from build123d import *

# Parameters (mm, degrees)
SKETCH1_W          = 5
SKETCH1_H          = 15
CLAMP_PART_DEPTH   = 2.5
SKETCH1_H_2        = 1.5
CLAMP_PART_2_DEPTH = 2.5
SKETCH2_R          = 1
OUTSIDE_DEPTH      = 2


with BuildPart() as part:
    # Sketch1 → Clamp part (new body)
    with BuildSketch(Plane(origin=(0, 0, -7), x_dir=(-1, 0, 0), z_dir=(0, 0, -1))):
        with Locations((19, 34)):
            Rectangle(SKETCH1_W, SKETCH1_H)
    extrude(amount=-CLAMP_PART_DEPTH)



with BuildPart() as body_2:
    # Sketch1 → Clamp part 2 (new body)
    with BuildSketch(Plane(origin=(0, 0, -7), x_dir=(-1, 0, 0), z_dir=(0, 0, -1))):
        with Locations((19, 17.25)):
            Rectangle(SKETCH1_W, SKETCH1_H_2)
    extrude(amount=-CLAMP_PART_2_DEPTH)


with BuildPart() as part_1:
    add(part.part)

    add(body_2.part)  # Outside merges body 2
    # Sketch2 → Outside (add)
    with BuildSketch(Plane(origin=(0, 0, -7), x_dir=(-1, 0, 0), z_dir=(0, 0, -1))):
        with BuildLine():
            Line((23.5, 43.5), (16.5, 43.5))
            Line((16.5, 43.5), (12.949489743, 43.5))
            ThreePointArc((12.949489743, 43.5), (10.5, 46.5), (8.050510257, 43.5))
            Line((8.050510257, 43.5), (-8.050510257, 43.5))
            ThreePointArc((-8.050510257, 43.5), (-10.5, 46.5), (-12.949489743, 43.5))
            Line((-12.949489743, 43.5), (-15.5, 43.5))
            Line((-15.5, 43.5), (-15.5, 41.5))
            Line((-15.5, 41.5), (16.5, 41.5))
            Line((16.5, 41.5), (16.5, 16.5))
            Line((16.5, 16.5), (11.5, 16.5))
            Line((11.5, 16.5), (11.5, 13.5))
            ThreePointArc((11.5, 13.5), (14, 11), (16.5, 13.5))
            Line((16.5, 13.5), (16.5, 14.5))
            Line((16.5, 14.5), (23.5, 14.5))
            Line((23.5, 14.5), (23.5, 43.5))
        make_face()
        with Locations((-10.5, 44)):
            Circle(SKETCH2_R, mode=Mode.SUBTRACT)
        with Locations((10.5, 44)):
            Circle(SKETCH2_R, mode=Mode.SUBTRACT)
        with Locations((14, 13.5)):
            Circle(SKETCH2_R, mode=Mode.SUBTRACT)
    extrude(amount=OUTSIDE_DEPTH)


solid = part_1.part
Geometry: final body of the model. Coordinates: model frame, mm. A direction names the side the tool comes from. Round coordinates to 2 decimals unless told otherwise and drop trailing zeros. Order: outer loops, then holes, each group sorted by start corner. A loop starts at its lowest first (then second) coordinate and runs counter-clockwise, first axis right, second up. Notation, with made-up numbers: (52, 44) - (100, 44) arc R30 ccw to (100, 77) - close; hole circle Ø1 at (36, 61.5). An arc over 180 degrees is marked (long way). Write each question's results on one line, items separated by ' | '.
Item 1: Section C-C, the plane y = 44. Return the cut outline in (x, z), and give its area (3 significant figures).
Completed:
outline: (-13, -9) - (-11.5, -9) - (-11.5, -7) - (-13, -7) - close; (-9.5, -9) - (-8, -9) - (-8, -7) - (-9.5, -7) - close; (8, -9) - (9.5, -9) - (9.5, -7) - (8, -7) - close; (11.5, -9) - (13, -9) - (13, -7) - (11.5, -7) - close | area: 12.0 mm^2
Item 2: Material intervals for line 1 along Y through (x, z) = (-14, -7.6); line 2 along Y through (x, z) = (-10.5, -7.45); line 3 along Y through (x, z) = (-21.5, -8.25), sorted ascending. Write a range as [from, to].
Completed:
line 1: [11, 12.5], [14.5, 16.5], [41.5, 43.5] | line 2: [41.5, 43], [45, 46.5] | line 3: [14.5, 43.5]
Item 3: Section D-D, the plane z = -7.55. Return the cut outline in (x, y).
Completed:
outline: (-23.5, 14.5) - (-16.5, 14.5) - (-16.5, 13.5) arc R2.5 ccw to (-11.5, 13.5) - (-11.5, 16.5) - (-16.5, 16.5) - (-16.5, 41.5) - (15.5, 41.5) - (15.5, 43.5) - (12.95, 43.5) arc R2.5 ccw (long way) to (8.05, 43.5) - (-8.05, 43.5) arc R2.5 ccw (long way) to (-12.95, 43.5) - (-23.5, 43.5) - close; hole circle Ø2 at (-14, 13.5); hole circle Ø2 at (-10.5, 44); hole circle Ø2 at (10.5, 44)
Item 4: Reachability of faces 1 (the flat face through (-19, 18, -6)), 2 (the flat face through (-16.5, 14, -8)), 3 (the flat face through (-14, 16.5, -8)), 4 (the flat face through (-11.5, 15, -8)), 5 (the flat face through (-21.5, 34, -6)) from +Z, -Z, +X, -X, +Y, -Y: full face, straight path, thin tool, end or side. Return the list, or none.
Completed:
face 1: +Z, +X, -X | face 2: +Z, -Z, -X, -Y | face 3: +Z, -Z, +X | face 4: +Z, -Z, +X, -Y | face 5: +Z, -X, +Y, -Y
Item 5: First-contact query: pin 1 Ø0.6 at (x, z) = (6, -7.5) entering from -Y; pin 2 Ø1.3 at (y, z) = (28.5, -6) entering from +X; pin 3 Ø0.5 at (y, z) = (14, -8) entering from -X; pin 4 Ø1.8 at (x, y) = (-10.5, 44) entering from -Z. Flat tips, straight axial feed; report the tip coordinate or a pass-through.
Completed:
pin 1: y = 41.5 | pin 2: x = -16.5 | pin 3: x = -16.5 | pin 4: through
Item 6: Section B-B, the plane x = -14. Return the cut outline in (y, z).
Completed:
outline: (11, -9) - (12.5, -9) - (12.5, -7) - (11, -7) - close; (14.5, -9) - (16.5, -9) - (16.5, -7) - (14.5, -7) - close; (41.5, -9) - (43.5, -9) - (43.5, -7) - (41.5, -7) - close
Item 7: Mould query, pull axis Y, two halves, no side actions, for faces 6 (the flat face through (-23.5, 29, -8)), 7 (the cylindrical face through (-10.37, 44.99, -7.99)), 8 (the flat face through (-20, 14.5, -8)). Classes: pulls with the +Y half, pulls with the -Y half, needs draft (parallel to the pull), parting line crosses it, or undercut.
Completed:
face 6: needs draft | face 7: undercut | face 8: pulls with the -Y half
Item 8: Section A-A, the plane z = -5.6. Return the cut outline in (x, y).
Completed:
outline: (-21.5, 16.5) - (-16.5, 16.5) - (-16.5, 18) - (-21.5, 18) - close; (-21.5, 26.5) - (-16.5, 26.5) - (-16.5, 41.5) - (-21.5, 41.5) - close
